from build123d import *

# Parameters (mm, degrees)
F0_R     = 3
F0_R_2   = 7
F1_DEPTH = 10
F2_W     = 200
F2_H     = 12
F3_DEPTH = 4.5
F4_W     = 200
F4_H     = 12
F5_DEPTH = 5
F6_R     = 5
F7_R     = 5
F8_R     = 5
F9_R     = 5
F10_R    = 5


with BuildPart() as f1:
    # F0 (on Top) → F1 (new body, symmetric)
    with BuildSketch(Plane.XY):
        Polygon((-40, 199.513814), (-60, 199.513814), (-60, -120.486186), (60, -120.486186), (60, 199.513814), (40, 199.513814), (40, -0.486186), (-40, -0.486186), align=None)
        with Locations((-12.5, -60.486186)):
            Circle(F0_R, mode=Mode.SUBTRACT)
        with Locations((0, -60.486186)):
            Circle(F0_R_2, mode=Mode.SUBTRACT)
        with Locations((12.5, -60.486186)):
            Circle(F0_R, mode=Mode.SUBTRACT)
    extrude(amount=F1_DEPTH, both=True)

    # F2 (on face) → F3 (join)
    with BuildSketch(Plane.YZ.offset(-40)):
        with Locations((99.513814, 0)):
            Rectangle(F2_W, F2_H)
    extrude(amount=F3_DEPTH)

    # F4 (on face) → F5 (join)
    with BuildSketch(Plane(origin=(40, 0, 0), x_dir=(0, -1, 0), z_dir=(-1, 0, 0))):
        with Locations((-99.513814, 0)):
            Rectangle(F4_W, F4_H)
    extrude(amount=F5_DEPTH)

    # F6
    f6_edges = [f1.edges().sort_by_distance(p)[0] for p in [
        (-60, 39.513814, 10),
    ]]
    fillet(f6_edges, radius=F6_R)

    # F7
    f7_edges = [f1.edges().sort_by_distance(p)[0] for p in [
        (-60, 39.513814, -10),
    ]]
    fillet(f7_edges, radius=F7_R)

    # F8
    f8_edges = [f1.edges().sort_by_distance(p)[0] for p in [
        (60, 39.513814, -10),
    ]]
    fillet(f8_edges, radius=F8_R)

    # F9
    f9_edges = [f1.edges().sort_by_distance(p)[0] for p in [
        (60, 39.513814, 10),
    ]]
    fillet(f9_edges, radius=F9_R)

    # F10
    f10_edges = [f1.edges().sort_by_distance(p)[0] for p in [
        (0, -120.486186, 10),
    ]]
    fillet(f10_edges, radius=F10_R)


solid = f1.part
The listing builds one solid part. Answer for the finished solid, in the listing's coordinates (mm). A direction names the side the tool comes from. Round coordinates to 2 decimals unless told otherwise and drop trailing zeros. Loops run counter-clockwise (first coordinate to the right, second up) from the corner with the lowest first, then second, coordinate; pieces in that order, holes last. Notation, with made-up numbers: M -33,44 L -29,44 A15 ccw -29,58 Z; hole C 69,7.5 d3. An arc over 180 degrees is marked long. Return JSON: item names as keys, results as strings.
Q1. Find section A-A, the plane y = 117.5. Determine the outline of the cut face in (x, z).
Results list:
{"outline": "M -60,-5 A5 ccw -55,-10 L -40,-10 L -40,-6 L -35.5,-6 L -35.5,6 L -40,6 L -40,10 L -55,10 A5 ccw -60,5 Z; M 35,-6 L 40,-6 L 40,-10 L 55,-10 A5 ccw 60,-5 L 60,5 A5 ccw 55,10 L 40,10 L 40,6 L 35,6 Z"}
Q2. Find section C-C, the plane z = -0.75. Determine the outline of the cut face in (x, y), plus the area to 3 significant figures.
Results list:
{"outline": "M -60,-115.49 A5 ccw -55,-120.49 L 55,-120.49 A5 ccw 60,-115.49 L 60,199.51 L 35,199.51 L 35,-0.49 L -35.5,-0.49 L -35.5,199.51 L -60,199.51 Z; hole C -12.5,-60.49 d6; hole C 0,-60.49 d14; hole C 12.5,-60.49 d6", "area": "24,100 mm2"}
Q3. Which of the six approach directions +Z, -Z, +X, -X, +Y, -Y give full straight-line access (tool end or side, diameter ignored) to faces 4 (the face through (35, 101, 0)), 5 (the face through (-1, -26, 10))?
Results list:
{"face 4": "+Z, -Z, +Y", "face 5": "+Z, +X, -X, +Y, -Y"}
Q4. The mould has two halves that part along X. Classify faces 1 (the face through (60, 40, 0)), 2 (the face through (-0.911, -53.546, -0.14)), 3 (the face through (48, 199.514, 0)): released by +X, released by -X, zero draft, split by the parting line, or undercut.
Results list:
{"face 1": "released by +X", "face 2": "undercut", "face 3": "zero draft"}
Q5. Find section B-B, the plane x = -12.5. Determine the outline of the cut face in (y, z).
Results list:
{"outline": "M -120.49,-5 A5 ccw -115.49,-10 L -63.49,-10 L -63.49,10 L -115.49,10 A5 ccw -120.49,5 Z; M -57.49,-10 L -0.49,-10 L -0.49,10 L -57.49,10 Z"}
Q6. Find section D-D, the plane x = 0. Determine the outline of the cut face in (y, z), plus the area to 3 significant figures.
Results list:
{"outline": "M -120.49,-5 A5 ccw -115.49,-10 L -67.49,-10 L -67.49,10 L -115.49,10 A5 ccw -120.49,5 Z; M -53.49,-10 L -0.49,-10 L -0.49,10 L -53.49,10 Z", "area": "2,110 mm2"}
Q7. Each of these flat-tipped pins is pushed along its axis until it touches: pin 1 Ø1.5 at (x, y) = (36.5, 68.5) entering from +Z; pin 2 Ø2 at (x, z) = (-7.5, 4.5) entering from +Y; pin 3 Ø2 at (y, z) = (132, -8) entering from -X. Where does it stop, or does it pass through?
Results list:
{"pin 1": "stops at z = 6", "pin 2": "stops at y = -0.49", "pin 3": "stops at x = -59.58"}
Q8. Find the intervals of material crossed by line 1 along Y through (x, z) = (12.5, 2.75); line 2 along Y through (x, z) = (-0.5, 4.25); line 3 along X through (y, z) = (179, -5.25), in increasing order. Write a range as from..to.
Results list:
{"line 1": "y = -120.49..-63.49, -57.49..-0.49", "line 2": "y = -120.49..-67.47, -53.5..-0.49", "line 3": "x = -59.99..-35.5, 35..59.99"}
